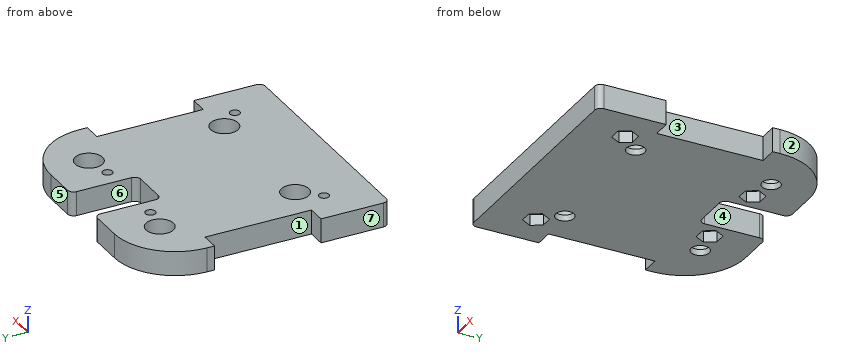
from build123d import *

# Parameters (mm, degrees)
SKETCH_1_W                   = 80
SKETCH_1_H                   = 80
EXTRUDE_1_DEPTH              = 8
SKETCH_7_W                   = 15
SKETCH_7_H                   = 22
CUT_EXTRUDE_1_DEPTH          = 10
HOLE_WIZARD_M4_1_D           = 3.3
HOLE_WIZARD_M4_1_CSINK_D     = 4.05
HOLE_WIZARD_M4_1_CSINK_ANGLE = 90
FILLET_1_R                   = 20
FILLET_2_R                   = 2
SKETCH_9_W                   = 6
SKETCH_9_H                   = 35
CUT_EXTRUDE_2_DEPTH          = 11
SKETCH_11_R                  = 3
CUT_EXTRUDE_4_DEPTH          = 15
CUT_EXTRUDE_5_DEPTH          = 3.6
SKETCH_13_R                  = 4.52
CUT_EXTRUDE_6_DEPTH          = 6


with BuildPart() as part:
    # 草图1 → 凸台-拉伸1 (new body)
    with BuildSketch(Plane.XY):
        Rectangle(SKETCH_1_W, SKETCH_1_H)
    extrude(amount=EXTRUDE_1_DEPTH)

    # 草图7 → 切除-拉伸1 (cut)
    with BuildSketch(Plane.XY.offset(8)):
        with Locations((0, 29)):
            Rectangle(SKETCH_7_W, SKETCH_7_H)
    extrude(amount=-CUT_EXTRUDE_1_DEPTH, mode=Mode.SUBTRACT)

    # M4 螺纹孔1 (through all)
    with Locations(Plane(origin=(13.5, 24.75, 0), x_dir=(-1, 0, 0), z_dir=(0, 0, -1))):
        with Locations((0, 0), (27, 0), (41.5, -49.5), (-14.5, -49.5)):
            CounterSinkHole(HOLE_WIZARD_M4_1_D / 2, HOLE_WIZARD_M4_1_CSINK_D / 2, counter_sink_angle=HOLE_WIZARD_M4_1_CSINK_ANGLE)

    # 圆角1
    fillet_1_edges = [part.edges().sort_by_distance(p)[0] for p in [
        (-40, 40, 4),
        (40, 40, 4),
    ]]
    fillet(fillet_1_edges, radius=FILLET_1_R)

    # 圆角2
    fillet_2_edges = [part.edges().sort_by_distance(p)[0] for p in [
        (-7.5, 18, 4),
        (-7.5, 40, 4),
        (7.5, 40, 4),
        (7.5, 18, 4),
        (40, -40, 4),
        (-40, -40, 4),
    ]]
    fillet(fillet_2_edges, radius=FILLET_2_R)

    # 草图9 → 切除-拉伸2 (cut)
    with BuildSketch(Plane.XY):
        with Locations((37, 0)):
            Rectangle(SKETCH_9_W, SKETCH_9_H)
        with Locations((-37, 0)):
            Rectangle(SKETCH_9_W, SKETCH_9_H)
    extrude(amount=CUT_EXTRUDE_2_DEPTH, mode=Mode.SUBTRACT)

    # 草图11 → 切除-拉伸4 (cut)
    with BuildSketch(Plane.XY):
        with Locations((-22.273863607, 26.273863607)):
            Circle(SKETCH_11_R)
        with Locations((22.273863607, 26.273863607)):
            Circle(SKETCH_11_R)
        with Locations((22.273863607, -18.273863607)):
            Circle(SKETCH_11_R)
        with Locations((-22.273863607, -18.273863607)):
            Circle(SKETCH_11_R)
    extrude(amount=CUT_EXTRUDE_4_DEPTH, mode=Mode.SUBTRACT)

    # 草图12 → 切除-拉伸5 (cut)
    with BuildSketch(Plane.XY):
        Polygon((11.531235582, 21.34), (15.468764418, 21.34), (17.437528836, 24.75), (15.468764418, 28.16), (11.531235582, 28.16), (9.562471164, 24.75), align=None)
        Polygon((26.031235582, -28.16), (29.968764418, -28.16), (31.937528836, -24.75), (29.968764418, -21.34), (26.031235582, -21.34), (24.062471164, -24.75), align=None)
        Polygon((-24.062471164, -24.75), (-26.031235582, -28.16), (-29.968764418, -28.16), (-31.937528836, -24.75), (-29.968764418, -21.34), (-26.031235582, -21.34), align=None)
        Polygon((-9.562471164, 24.75), (-11.531235582, 21.34), (-15.468764418, 21.34), (-17.437528836, 24.75), (-15.468764418, 28.16), (-11.531235582, 28.16), align=None)
    extrude(amount=CUT_EXTRUDE_5_DEPTH, mode=Mode.SUBTRACT)

    # 草图13 → 切除-拉伸6 (cut)
    with BuildSketch(Plane.XY.offset(8)):
        with Locations((-22.273863607, 26.273863607)):
            Circle(SKETCH_13_R)
        with Locations((-22.273863607, -18.273863607)):
            Circle(SKETCH_13_R)
        with Locations(Location((22.273863607, -18.273863607, 0), (0, 0, 180))):
            Circle(SKETCH_13_R)
        with Locations(Location((22.273863607, 26.273863607, 0), (0, 0, 180))):
            Circle(SKETCH_13_R)
    extrude(amount=-CUT_EXTRUDE_6_DEPTH, mode=Mode.SUBTRACT)


solid = part.part
Design review of the part built by this model. Coordinates are the model's own, in mm. Face numbers are marked on the shaded views. A direction names the side the tool comes from. Give positions to 0.01 mm unless a question says otherwise; leave off trailing zeros. Order: outer loops, then holes, each group sorted by start corner. A loop starts at its lowest first (then second) coordinate and runs counter-clockwise, first axis right, second up. Notation, with made-up numbers: (78, 73.25) - (114, 73.25) arc R23 cw to (114, 101.25) - close; hole circle Ø2 at (12, -8). An arc over 180 degrees is marked (long way). Write item = value, one per line. Start each with the question number.
Q1. We need section B-B on y = -20. State the section outline as (x, z) points.
Q2. We need section A-A on x = 13.5. State the section outline as (y, z) points, plus the area to 3 significant figures.
Q3. We need section D-D on x = -35. State the section outline as (y, z) points, plus the area to 3 significant figures.
Q4. We need section C-C on z = 5. State how many separate pieces and enclosed holes the cut face has, plus the area to 3 significant figures.
Q5. Tool access review of the marked faces 1, 2 and 3: name each direction out of +Z, -Z, +X, -X, +Y, -Y from which nothing blocks a thin tool from reaching the whole face with its end or side.
Q6. To check wall thickness, follow L1, parallel to Y at x = 22.5, z = 6.5; L2, parallel to Y at x = -19, z = 2.5; L3, parallel to Z at x = -28.5, y = -23. State the ranges of each line that lie inside material, in increasing order. Write a range as from..to.
Q7. Mouldability with a two-part tool opening along X and no side actions: class the marked faces 4, 5, 6 and 7 as released by +X, released by -X, zero draft, split by the parting line, or undercut.
Q8. Clearance check with flat-ended pins moving along their axes: pin 1 Ø4.5 at (x, y) = (-13.5, 24.75) entering from -Z; pin 2 Ø3 at (x, z) = (26, 2.5) entering from +Y. State where each tip first meets the part, or that it passes through.
Working result:
q1.outline = (-40, 0) - (-24.73, 0) - (-24.73, 2) - (-26.45, 2) - (-26.45, 8) - (-40, 8) - close; (-19.82, 0) - (19.82, 0) - (19.82, 2) - (18.1, 2) - (18.1, 8) - (-18.1, 8) - (-18.1, 2) - (-19.82, 2) - close; (24.73, 0) - (40, 0) - (40, 8) - (26.45, 8) - (26.45, 2) - (24.73, 2) - close
q2.outline = (-40, 0) - (21.34, 0) - (21.34, 3.6) - (23.1, 3.6) - (23.1, 8) - (-40, 8) - close; (26.4, 3.6) - (28.16, 3.6) - (28.16, 0) - (40, 0) - (40, 8) - (26.4, 8) - close
q2.area = 601 mm²
q3.outline = (-40, 0) - (-17.5, 0) - (-17.5, 8) - (-40, 8) - close; (17.5, 0) - (33.23, 0) - (33.23, 8) - (17.5, 8) - close
q3.area = 306 mm²
q4.separate_pieces = 1
q4.enclosed_holes = 8
q4.area = 5,190 mm²
q5.face_1 = +Z, -Z, -X
q5.face_2 = +Z, -Z, +X, +Y
q5.face_3 = +Z, -Z, +X
q6.L1 = -40..-22.79, -13.76..21.76, 30.79..39.84
q6.L2 = -40..-21.39, -15.16..23.16, 29.39..40
q6.L3 = 3.6..8
q7.face_4 = undercut
q7.face_5 = zero draft
q7.face_6 = undercut
q7.face_7 = released by -X
q8.pin_1 = 3.6
q8.pin_2 = 39.49
